```python
from build123d import *

# Parameters (mm, degrees)
SKETCH1_W           = 15
SKETCH1_H           = 9
BOSS_EXTRUDE1_DEPTH = 15
BOSS_EXTRUDE3_START = 2
BOSS_EXTRUDE3_DEPTH = 2
SKETCH7_W           = 15
SKETCH7_H           = 9
BOSS_EXTRUDE4_DEPTH = 15
FILLET1_R           = 1
CHAMFER1_SIZE       = 2.5


with BuildPart() as part:
    # Sketch1 → Boss-Extrude1 (new body)
    with BuildSketch(Plane.XY):
        with BuildLine():
            ThreePointArc((0, -17.5), (12.374368671, -12.374368671), (17.5, 0))
            Line((17.5, 0), (11, 0))
            ThreePointArc((11, 0), (7.778174593, -7.778174593), (0, -11))
            Line((0, -11), (0, -17.5))
        make_face()
        with BuildLine():
            ThreePointArc((-17.5, 0), (-12.374368671, -12.374368671), (0, -17.5))
            Line((0, -17.5), (0, -11))
            ThreePointArc((0, -11), (-7.778174593, -7.778174593), (-11, 0))
            Line((-11, 0), (-17.5, 0))
        make_face()
        with BuildLine():
            ThreePointArc((-4.25, 16.976086121), (-13.795379661, 10.767427734), (-17.5, 0))
            Line((-17.5, 0), (-11, 0))
            ThreePointArc((-11, 0), (-9.158329542, 6.093028803), (-4.25, 10.145811944))
            Line((-4.25, 10.145811944), (-4.25, 16.976086121))
        make_face()
        with BuildLine():
            Line((11, 0), (17.5, 0))
            ThreePointArc((17.5, 0), (13.795379661, 10.767427734), (4.25, 16.976086121))
            Line((4.25, 16.976086121), (4.25, 10.145811944))
            ThreePointArc((4.25, 10.145811944), (9.158329542, 6.093028803), (11, 0))
        make_face()
        with BuildLine():
            Line((8.5, -71), (17.5, -30))
            Line((17.5, -30), (8.5, -30))
            Line((8.5, -30), (-0.5, -71))
            Line((-0.5, -71), (-8.5, -71))
            Line((-8.5, -71), (-8.5, -17.5))
            Line((-8.5, -17.5), (0, -17.5))
            ThreePointArc((0, -17.5), (-12.374368671, -12.374368671), (-17.5, 0))
            Line((-17.5, 0), (-17.5, -71))
            Line((-17.5, -71), (-17.5, -80))
            Line((-17.5, -80), (8.5, -80))
            Line((8.5, -80), (8.5, -71))
        make_face()
        with BuildLine():
            Line((17.5, -30), (17.5, 0))
            ThreePointArc((17.5, 0), (12.374368671, -12.374368671), (0, -17.5))
            Line((0, -17.5), (8.5, -17.5))
            Line((8.5, -17.5), (8.5, -30))
            Line((8.5, -30), (17.5, -30))
        make_face()
        with Locations((-25, -75.5)):
            Rectangle(SKETCH1_W, SKETCH1_H)
    extrude(amount=BOSS_EXTRUDE1_DEPTH)

    # Sketch6 → Boss-Extrude3 (add)
    with BuildSketch(Plane(origin=(0, 0, 15), x_dir=(-1, 0, 0), z_dir=(0, 0, -1)).offset(BOSS_EXTRUDE3_START)):
        with BuildLine():
            Line((-4.25, 7.933315826), (-4.25, 10.145811944))
            ThreePointArc((-4.25, 10.145811944), (-6.093028803, -9.158329542), (11, 0))
            ThreePointArc((11, 0), (9.158329542, 6.093028803), (4.25, 10.145811944))
            Line((4.25, 10.145811944), (4.25, 7.933315826))
            ThreePointArc((4.25, 7.933315826), (7.721722606, 4.623310502), (9, 0))
            ThreePointArc((9, 0), (-4.623310502, -7.721722606), (-4.25, 7.933315826))
        make_face()
    extrude(amount=-BOSS_EXTRUDE3_DEPTH)

    # Sketch7 → Boss-Extrude4 (add)
    with BuildSketch(Plane.XY.offset(15)):
        with Locations((1, -75.5)):
            Rectangle(SKETCH7_W, SKETCH7_H)
    extrude(amount=BOSS_EXTRUDE4_DEPTH)

    # Sketch11 → Cut-Revolve4 (revolve, cut)
    with BuildSketch(Plane.ZY.offset(25)):
        Polygon((7.5, -71), (7.5, -80), (9.7, -80), (9.7, -74), (12.307860213, -71), align=None)
    revolve(axis=Axis((-25, -71, 7.5), (0, -1, 0)), mode=Mode.SUBTRACT)

    # Sketch10 → Cut-Revolve3 (revolve, cut)
    with BuildSketch(Plane.XY.offset(22.5), mode=Mode.PRIVATE) as cut_revolve3_sk:
        Polygon((1, -71), (5.807860213, -71), (3.2, -74), (3.2, -80), (1, -80), align=None)
    revolve(cut_revolve3_sk.sketch.rotate(Axis((1, -80, 22.5), (0, 1, 0)), 90), axis=Axis((1, -80, 22.5), (0, 1, 0)), mode=Mode.SUBTRACT)

    # Fillet1
    fillet1_edges = [part.edges().sort_by_distance(p)[0] for p in [
        (0, -11, 0),
    ]]
    fillet(fillet1_edges, radius=FILLET1_R)

    # Chamfer1
    chamfer1_edges = [part.edges().sort_by_distance(p)[0] for p in [
        (-32.5, -75.5, 0),
        (-8.5, -17.5, 7.5),
        (8.5, -17.5, 7.5),
        (-32.5, -75.5, 15),
        (-6.5, -75.5, 30),
        (8.5, -75.5, 30),
    ]]
    chamfer(chamfer1_edges, length=CHAMFER1_SIZE)


solid = part.part
```
Work out the finished part from the listing and answer in its coordinate system (mm). A direction names the side the tool comes from. Give positions to 0.01 mm unless a question says otherwise; leave off trailing zeros. Loops run counter-clockwise (first coordinate to the right, second up) from the corner with the lowest first, then second, coordinate; pieces in that order, holes last. Notation, with made-up numbers: (51.5, -21) - (65.5, -21) arc R17 ccw to (65.5, -17) - close; hole circle Ø9 at (-4.75, 87). An arc over 180 degrees is marked (long way). Use CSV: the item, a comma, the result in double quotes. Start each with the question number.
(1) Find section B-B, the plane y = -28. Determine the outline of the cut face in (x, z), plus the area to 3 significant figures.
(2) Each of these flat-tipped pins is pushed along its axis until it touches: pin 1 (20.5 mm diameter, centred on x = 0, y = 0, fed in from +Z); pin 2 (13.5 mm diameter, centred on x = -1.5, z = 22, fed in from +Y); pin 3 (8 mm diameter, centred on y = -26.5, z = 8, fed in from -X). Where does it stop, or does it pass through?
(3) Find section C-C, the plane x = 2. Count the separate pieces of the cut face and the enclosed holes in it, plus the area to 3 significant figures.
(4) A tool of negligible diameter and unlimited length cuts with its end or side. For faces 1 (the face through (-2, -71, 15)), 2 (the face through (-8.5, -46, 7)), 3 (the face through (-20, -71, 7)), 4 (the face through (8.5, -76, 14)), 5 (the face through (4.25, 13, 7)), from which of +Z, -Z, +X, -X, +Y, -Y can it reach the whole face along a straight path? Write none if from no direction.
(5) Find the intervals of material crossed by L1, parallel to Y at x = -5.5, z = 9; L2, parallel to Y at x = -3, z = 13.5; L3, parallel to Z at x = 15, y = -31, in increasing order.
(6) Determine the mould class of faces 6 (the face through (-22.852, -76.958, 7.023)), 7 (the face through (-31, -76, 1)), 8 (the face through (7.3, -18.8, 7.4)) for opening direction Z: released by +Z, released by -Z, zero draft, split by the parting line, or undercut.
(7) Find section A-A, the plane z = 22.5. Determine the outline of the cut face in (x, y).
Results found:
1,outline,"(-17.5, 0) - (-8.5, 0) - (-8.5, 15) - (-17.5, 15) - close; (8.5, 0) - (17.5, 0) - (17.5, 15) - (8.5, 15) - close"
1,area,"270 mm^2"
2,pin 1,"z = 15"
2,pin 2,"y = -71"
2,pin 3,"x = -17.5"
3,separate pieces,"3"
3,enclosed holes,"0"
3,area,"501 mm^2"
4,face 1,"+Z"
4,face 2,"+Z, -Z"
4,face 3,"+Z, -Z, -X, +Y"
4,face 4,"+Z, -Z, +X, -Y"
4,face 5,"+Z, -Z, +Y"
5,L1,"-80 to -71, -17.5 to -9.53, 9.53 to 16.61"
5,L2,"-80 to -71, -17.5 to -8.49"
5,L3,"0 to 15"
6,face 6,"undercut"
6,face 7,"released by -Z"
6,face 8,"zero draft"
7,outline,"(-6.5, -80) - (-1.2, -80) - (-1.2, -74) - (-3.81, -71) - (-6.5, -71) - close; (3.2, -80) - (8.5, -80) - (8.5, -71) - (5.81, -71) - (3.2, -74) - close"
